from build123d import *

# Parameters (mm, degrees)
F0_R     = 23
F0_R_2   = 20
F1_DEPTH = 5
F0_R_3   = 26
F2_DEPTH = 5
F3_R     = 3.175
F4_SIZE  = 1.27
F5_SIZE  = 1.016


with BuildPart() as f1:
    # F0 (on Top) → F1 (new body)
    with BuildSketch(Plane.XY):
        Circle(F0_R)
        Circle(F0_R_2, mode=Mode.SUBTRACT)
    extrude(amount=F1_DEPTH)

    # F0 (on Top) → F2 (join)
    with BuildSketch(Plane.XY):
        Circle(F0_R_3)
        Circle(F0_R, mode=Mode.SUBTRACT)
    extrude(amount=F2_DEPTH)

    # F3
    f3_edges = [f1.edges().sort_by_distance(p)[0] for p in [
        (-26, 0, 5),
    ]]
    fillet(f3_edges, radius=F3_R)

    # F4
    f4_edges = [f1.edges().sort_by_distance(p)[0] for p in [
        (-20, 0, 5),
    ]]
    chamfer(f4_edges, length=F4_SIZE)

    # F5
    f5_edges = [f1.edges().sort_by_distance(p)[0] for p in [
        (-26, 0, 0),
    ]]
    chamfer(f5_edges, length=F5_SIZE)


solid = f1.part
Input: part model. Units: mm. Frame: model coordinates. Give positions to 0.01 mm unless a question says otherwise; leave off trailing zeros. Write each loop counter-clockwise with the first axis right and the second up, starting at its lowest first coordinate (ties: lowest second). Pieces come first, ordered by that corner, then holes. Notation, with made-up numbers: M -0.5,-17.5 L 52.5,-17.5 A15 ccw 52.5,5.5 Z; hole C 18.5,46 d6. An arc over 180 degrees is marked long. Write item = value, one per line. Start each with the question number.
1) Cut plane C-C on z = 3.1. Return the cut outline in (x, y), then the cut area to 3 significant figures.
2) Cut plane A-A on y = 0. Return the cut outline in (x, z) (3 decimals), then the cut area to 3 significant figures.
3) First-contact query: pin 1 Ø2 at (x, z) = (12, 2) entering from +Y; pin 2 Ø3 at (x, z) = (-10.5, 1) entering from -Y; pin 3 Ø2 at (y, z) = (17, 1) entering from +X; pin 4 Ø5 at (x, y) = (5, -19) entering from -Z. Flat tips, straight axial feed; report the tip coordinate or a pass-through.
4) Draft query along X for faces 1 (the cylindrical face through (-4.336, -19.524, 1.839)), 2 (the cylindrical face through (-20.633, -15.821, 1.415)), 3 (the flat face through (-19, 10, 5)). Return one class per face: +X half, -X half, draft (parallel to the pull), parting line (faces both ways), or undercut.
5) Material intervals for line 1 along Y through (x, z) = (0, 1.1); line 2 along X through (y, z) = (1, 2.1); line 3 along X through (y, z) = (-0.5, 0.2), sorted ascending. Write a range as [from, to].
Solved:
q1.outline = C 0,0 d51.47; hole C 0,0 d40
q1.area = 824 mm2
q2.outline = M -26,1.016 L -24.984,0 L -20,0 L -20,3.73 L -21.27,5 L -22.825,5 A3.175 ccw -26,1.825 Z; M 20,0 L 24.984,0 L 26,1.016 L 26,1.825 A3.175 ccw 22.825,5 L 21.27,5 L 20,3.73 Z
q2.area = 53.0 mm2
q3.pin_1 = 23.56
q3.pin_2 = -24.39
q3.pin_3 = 20.49
q3.pin_4 = 0
q4.face_1 = undercut
q4.face_2 = parting line
q4.face_3 = draft
q5.line_1 = [-26, -20], [20, 26]
q5.line_2 = [-25.97, -19.97], [19.97, 25.97]
q5.line_3 = [-25.18, -19.99], [19.99, 25.18]
